```python
from build123d import *

# Parameters (mm, degrees)
F0_W     = 259.929892
F0_H     = 140
F0_W_2   = 260
F0_W_3   = 500
F2_DEPTH = 600
F3_DEPTH = 2
F4_W     = 60
F4_H     = 60
F5_W     = 60
F5_H     = 60
F6_DEPTH = 370
F6_TAPER = 1.5


with BuildPart() as f2:
    # F0 (on Front) → F2 (new body)
    with BuildSketch(Plane.XZ):
        Polygon((550, 172.5), (-550, 172.5), (-550, -172.5), (-500.11901, -172.5), (-250, -172.5), (-250, -12.5), (250, -12.5), (250, -172.5), (490, -172.5), (550, -172.5), align=None)
        with Locations((-400.035054, -82.5)):
            Rectangle(F0_W, F0_H, mode=Mode.SUBTRACT)
        with Locations((400, -82.5)):
            Rectangle(F0_W_2, F0_H, mode=Mode.SUBTRACT)
        with Locations((-400, 77.5)):
            Rectangle(F0_W_2, F0_H, mode=Mode.SUBTRACT)
        with Locations((0, 77.5)):
            Rectangle(F0_W_3, F0_H, mode=Mode.SUBTRACT)
        with Locations((400, 77.5)):
            Rectangle(F0_W_2, F0_H, mode=Mode.SUBTRACT)
    extrude(amount=F2_DEPTH)

    # F1 (on Front) → F3 (join)
    with BuildSketch(Plane.XZ):
        Polygon((550, -172.5), (550, 172.5), (-550, 172.5), (-550, -172.5), (-250, -172.5), (-250, -12.5), (250, -12.5), (250, -172.5), align=None)
    extrude(amount=-F3_DEPTH)

    # F4 (on face) + F5 (on face) → F6 (join)
    with BuildSketch(Plane(origin=(0, 0, -172.5), x_dir=(1, 0, 0), z_dir=(0, 0, -1))):
        with Locations((-520, 570)):
            Rectangle(F4_W, F4_H)
        with Locations((-520, 30)):
            Rectangle(F4_W, F4_H)
    with BuildSketch(Plane(origin=(0, 0, -172.5), x_dir=(1, 0, 0), z_dir=(0, 0, -1))):
        with Locations((520, 570)):
            Rectangle(F5_W, F5_H)
        with Locations((520, 30)):
            Rectangle(F5_W, F5_H)
    extrude(amount=F6_DEPTH, taper=F6_TAPER)


solid = f2.part
```
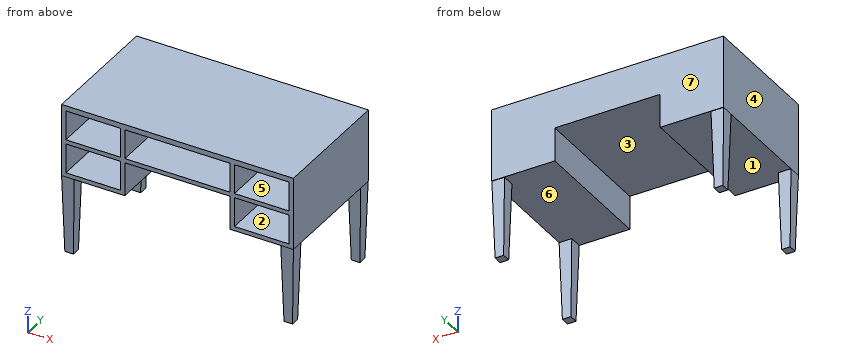
Can you work these out from the model? Positions are in its coordinate system, mm. Face numbers are marked on the shaded views. A direction names the side the tool comes from. Coordinates: 2 decimals unless noted, no trailing zeros. Loops run counter-clockwise (first coordinate to the right, second up) from the corner with the lowest first, then second, coordinate; pieces in that order, holes last. Notation, with made-up numbers: (-13, 82.25) -> (11, 82.25) arc R14 ccw to (11, 97.25) -> close; hole circle Ø4 at (-24.5, -16). An arc over 180 degrees is marked (long way). Put each result on its own line as item: value. Start each with the question number.
Q1. I'm going to push a flat-ended pin straight in: P1, Ø6, axis at x = -339, y = -61.5, coming from the -Z side. Where does the tip first touch, or does it pass through?
Q2. I want a section at B-B (x = -137). Write out the boundary of the cut face in (y, z), plus the area to 3 significant figures.
Q3. If I drill on line 1 (Z direction, x = 485, y = -212); line 2 (X direction, y = -379.5, z = 110); line 3 (X direction, y = -436, z = -55), over which ranges is the centre line in solid material (lowest first)? Write a range as [from, to].
Q4. I want a section at A-A (y = -446). Write out the boundary of the cut face in (x, z).
Q5. I want a section at C-C (z = 22). Write out the boundary of the cut face in (x, y).
Q6. Thinking about a two-plate mould opening in Y: for the marked faces 5, 6 and 7, which applies, pulls with the +Y half, pulls with the -Y half, needs draft (parallel to the pull), parting line crosses it, or undercut?
Q7. For the marked faces 1, 2, 3 and 4, which set-ups out of +Z, -Z, +X, -X, +Y, -Y let a thin tool reach every point of the face, with its end or its side?
Q8. I want a section at D-D (x = 335.5). Write out the boundary of the cut face in (y, z).
Taken from the geometry:
1. P1: stops at z = -172.5
2. outline: (-600, -12.5) -> (2, -12.5) -> (2, 172.5) -> (-600, 172.5) -> (-600, 147.5) -> (0, 147.5) -> (0, 7.5) -> (-600, 7.5) -> close
2. area: 27,400 mm2
3. line 1: z = [-172.5, -152.5], [-12.5, 7.5], [147.5, 172.5]
3. line 2: x = [-550, -530], [-270, -250], [250, 270], [530, 550]
3. line 3: x = [-550, -530], [-270.07, -250], [250, 270], [530, 550]
4. outline: (-550, -172.5) -> (-250, -172.5) -> (-250, -12.5) -> (250, -12.5) -> (250, -172.5) -> (550, -172.5) -> (550, 172.5) -> (-550, 172.5) -> close; hole (-530, -152.5) -> (-270.07, -152.5) -> (-270.07, -12.5) -> (-530, -12.5) -> close; hole (-530, 7.5) -> (-270, 7.5) -> (-270, 147.5) -> (-530, 147.5) -> close; hole (-250, 7.5) -> (250, 7.5) -> (250, 147.5) -> (-250, 147.5) -> close; hole (270, -152.5) -> (530, -152.5) -> (530, -12.5) -> (270, -12.5) -> close; hole (270, 7.5) -> (530, 7.5) -> (530, 147.5) -> (270, 147.5) -> close
5. outline: (-550, -600) -> (-530, -600) -> (-530, 0) -> (-270, 0) -> (-270, -600) -> (-250, -600) -> (-250, 0) -> (250, 0) -> (250, -600) -> (270, -600) -> (270, 0) -> (530, 0) -> (530, -600) -> (550, -600) -> (550, 2) -> (-550, 2) -> close
6. face 5: needs draft
6. face 6: undercut
6. face 7: pulls with the +Y half
7. face 1: -Z
7. face 2: -Y
7. face 3: -Z, +Y, -Y
7. face 4: +Z, -Z, -X, +Y, -Y
8. outline: (-600, -172.5) -> (2, -172.5) -> (2, 172.5) -> (-600, 172.5) -> (-600, 147.5) -> (0, 147.5) -> (0, 7.5) -> (-600, 7.5) -> (-600, -12.5) -> (0, -12.5) -> (0, -152.5) -> (-600, -152.5) -> close
